CAD build for the part. Positions are in the model's coordinates, mm. A direction names the side the tool comes from. Round coordinates to 2 decimals unless told otherwise and drop trailing zeros. Write each loop counter-clockwise with the first axis right and the second up, starting at its lowest first coordinate (ties: lowest second). Pieces come first, ordered by that corner, then holes. Notation, with made-up numbers: (25.5, 30) - (40.5, 30) arc R17 ccw to (40.5, 51) - close; hole circle Ø8 at (-38, 86.5). An arc over 180 degrees is marked (long way). Put each result on its own line as item: value. Start each with the question number.
Item 1: Cut at B-B (z = 0). Give the cut face in (x, y).
Item 2: Drill centre lines: line 1 (X direction, y = 1.5, z = -10.1); line 2 (X direction, y = 50, z = 0); line 3 (Z direction, x = -20, y = 2). Where is each one in solid material? Low to high. Write a range as from..to.
Item 3: Cut at A-A (x = -27.7). Give the cut face in (y, z).
Item 4: 3-axis set-ups, long thin cutter, end or side, ignore diameter. For faces 4 (the flat face through (-10, 44.8, 0)), 5 (the flat face through (21, 3, -10)), 6 (the flat face through (-22.5, 41, 0)), 7 (the flat face through (-31, 34, 1.381)), 8 (the flat face through (22.5, 15, 0)): which of +Z, -Z, +X, -X, +Y, -Y reach the whole face in a straight line?
Item 5: Pin check, flat tips, straight feed: pin 1 Ø0.9 at (x, z) = (-21, 10) entering from -Y; pin 2 Ø5 at (x, z) = (20.5, 10.1) entering from +Y; pin 3 Ø1.5 at (y, z) = (22.5, -9) entering from -X. Stop position of each tip, or through.
Item 6: Cut at D-D (y = 48.5). Give the cut face in (x, z).
Item 7: Cut at C-C (x = 20.5). Give the cut face in (y, z), and give its area (3 significant figures).
Item 8: Mould opens along Z. For faces 1 (the flat face through (-32.3, 34, 7)), 2 (the flat face through (31, 34, 1.381)), 3 (the cylindrical face through (-22.39, 49.04, -0.46)) say: released by +Z, released by -Z, zero draft, split by the parting line, or undercut.
```python
from build123d import *

# Parameters (mm, degrees)
SKETCH1_W           = 45
SKETCH1_H           = 24.2
BOSS_EXTRUDE1_DEPTH = 44.8
SKETCH2_W           = 24.2
SKETCH2_H           = 5
BOSS_EXTRUDE2_DEPTH = 9.8
CUT_EXTRUDE1_DEPTH  = 51.146385712
SKETCH4_R           = 4.86
BOSS_EXTRUDE3_DEPTH = 8.6
SKETCH5_R           = 1.5
CUT_EXTRUDE2_DEPTH  = 3


with BuildPart() as part:
    # Sketch1 → Boss-Extrude1 (new body)
    with BuildSketch(Plane(origin=(0, 0, 0), x_dir=(1, 0, 0), z_dir=(0, 1, 0))):
        Rectangle(SKETCH1_W, SKETCH1_H)
    extrude(amount=BOSS_EXTRUDE1_DEPTH)

    # Sketch2 → Boss-Extrude2 (add)
    with BuildSketch(Plane.ZY.offset(22.5)):
        with Locations((0, 33.9)):
            Rectangle(SKETCH2_W, SKETCH2_H)
    boss_extrude2 = extrude(amount=BOSS_EXTRUDE2_DEPTH)

    # Sketch3 → Cut-Extrude1 (cut, symmetric)
    with BuildSketch(Plane(origin=(0, 36.4, 0), x_dir=(1, 0, 0), z_dir=(0, 1, 0))):
        with BuildLine():
            Line((-29.412527121, 1.381032534), (-32.3, 1.381032534))
            Line((-32.3, 1.381032534), (-32.3, -1.381032534))
            Line((-32.3, -1.381032534), (-29.412527121, -1.381032534))
            ThreePointArc((-29.412527121, -1.381032534), (-25.5, 0), (-29.412527121, 1.381032534))
        make_face()
    cut_extrude1 = extrude(amount=CUT_EXTRUDE1_DEPTH, both=True, mode=Mode.SUBTRACT)

    # Mirror2: Boss-Extrude2, Cut-Extrude1 across plane
    add(boss_extrude2.mirror(Plane.ZY))
    add(cut_extrude1.mirror(Plane.ZY), mode=Mode.SUBTRACT)

    # Sketch4 → Boss-Extrude3 (add)
    with BuildSketch(Plane(origin=(0, 44.8, 0), x_dir=(1, 0, 0), z_dir=(0, 1, 0))):
        with BuildLine():
            ThreePointArc((0.686331497, 5.070554234), (-22.4, 0), (0.686331497, -5.070554234))
            ThreePointArc((0.686331497, -5.070554234), (8.316936989, 0), (0.686331497, 5.070554234))
        make_face()
        with Locations(Location((-10.3, 0, 0), (0, 0, 90))):
            Circle(SKETCH4_R, mode=Mode.SUBTRACT)
    extrude(amount=BOSS_EXTRUDE3_DEPTH)

    # Sketch5 → Cut-Extrude2 (cut)
    with BuildSketch(Plane.XZ):
        with Locations(Location((-20.5, 10.1, 0), (0, 0, 270))):
            Circle(SKETCH5_R)
        with Locations(Location((20.5, 10.1, 0), (0, 0, 270))):
            Circle(SKETCH5_R)
        with Locations(Location((20.5, -10.1, 0), (0, 0, 270))):
            Circle(SKETCH5_R)
        with Locations(Location((-20.5, -10.1, 0), (0, 0, 270))):
            Circle(SKETCH5_R)
    extrude(amount=-CUT_EXTRUDE2_DEPTH, mode=Mode.SUBTRACT)


solid = part.part
```
Output values:
1. outline: (-25.5, 31.4) - (-22.5, 31.4) - (-22.5, 0) - (22.5, 0) - (22.5, 31.4) - (25.5, 31.4) - (25.5, 36.4) - (22.5, 36.4) - (22.5, 44.8) - (8.32, 44.8) - (8.32, 53.4) - (-5.44, 53.4) - (-5.44, 44.8) - (-15.16, 44.8) - (-15.16, 53.4) - (-22.4, 53.4) - (-22.4, 44.8) - (-22.5, 44.8) - (-22.5, 36.4) - (-25.5, 36.4) - close
2. line 1: -22.5..-22, -19..19, 22..22.5
2. line 2: -22.4..-15.16, -5.44..8.32
2. line 3: -12.1..-11.51, -8.69..8.69, 11.51..12.1
3. outline: (31.4, -12.1) - (36.4, -12.1) - (36.4, -2.2) - (31.4, -2.2) - close; (31.4, 2.2) - (36.4, 2.2) - (36.4, 12.1) - (31.4, 12.1) - close
4. face 4: +Y
4. face 5: -Y
4. face 6: +Z, -Z, -X, +Y
4. face 7: -X, +Y, -Y
4. face 8: +Z, -Z, +X, -Y
5. pin 1: y = 3
5. pin 2: y = 44.8
5. pin 3: x = -22.5
6. outline: (0.69, -5.07) arc R5.5 ccw (long way) to (0.69, 5.07) arc R12.1 ccw (long way) to start; hole circle Ø9.72 at (-10.3, 0)
7. outline: (0, -12.1) - (44.8, -12.1) - (44.8, 12.1) - (0, 12.1) - (0, 11.6) - (3, 11.6) - (3, 8.6) - (0, 8.6) - (0, -8.6) - (3, -8.6) - (3, -11.6) - (0, -11.6) - close
7. area: 1,070 mm2
8. face 1: zero draft
8. face 2: undercut
8. face 3: split by the parting line
